Here's how the part is built. I have some questions about the finished solid (model axes, mm). Give positions to 0.01 mm unless a question says otherwise; leave off trailing zeros. Loops run counter-clockwise (first coordinate to the right, second up) from the corner with the lowest first, then second, coordinate; pieces in that order, holes last.
Q1. I need wall thicknesses on line 1 (X direction, y = 6.75, z = 0); line 2 (Z direction, x = 200, y = 12); line 3 (Z direction, x = 107, y = 14.25). Which ranges of each line are inside material? Lowest first, please.
Q2. If we section it at B-B (x = 59.5): Please give me the cut outline in (y, z), plus the area to 3 significant figures.
Q3. If we section it at C-C (y = 13): Please give me the cut outline in (x, z), plus the area to 3 significant figures.
Q4. If we section it at A-A (z = -12.5): Please give me the cut outline in (x, y).
Q5. Will this pin go through, and if not, where does the flat tip stop? P1, Ø12, axis at x = -284.5, z = 59.5, coming from the -Y side.
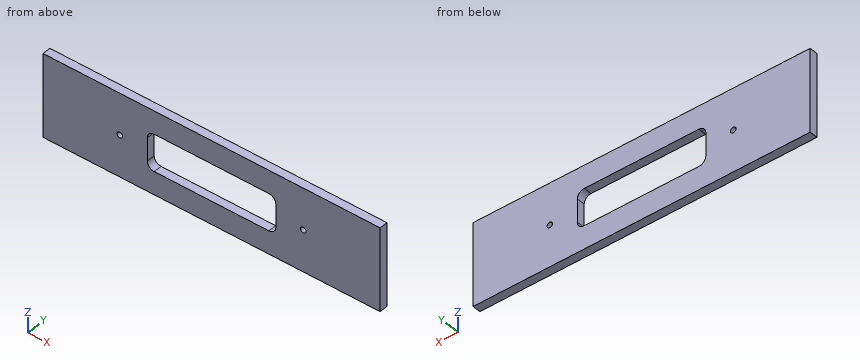
from build123d import *

# Parameters (mm, degrees)
SKETCH1_W           = 735
SKETCH1_H           = 180
BOSS_EXTRUDE1_DEPTH = 18
SKETCH2_R           = 6
CUT_EXTRUDE1_DEPTH  = 60


with BuildPart() as part:
    # Sketch1 → Boss-Extrude1 (new body)
    with BuildSketch(Plane(origin=(0, 0, 0), x_dir=(1, 0, 0), z_dir=(0, 1, 0))):
        Rectangle(SKETCH1_W, SKETCH1_H)
    extrude(amount=BOSS_EXTRUDE1_DEPTH)

    # Sketch2 → Cut-Extrude1 (cut)
    with BuildSketch(Plane(origin=(0, 18, 0), x_dir=(1, 0, 0), z_dir=(0, 1, 0))):
        with Locations((-200, 0)):
            Circle(SKETCH2_R)
        with Locations((200, 0)):
            Circle(SKETCH2_R)
        with BuildLine():
            Line((-125, -40), (125, -40))
            ThreePointArc((125, -40), (135.606601718, -35.606601718), (140, -25))
            Line((140, -25), (140, 25))
            ThreePointArc((140, 25), (135.606601718, 35.606601718), (125, 40))
            Line((125, 40), (-125, 40))
            ThreePointArc((-125, 40), (-135.606601718, 35.606601718), (-140, 25))
            Line((-140, 25), (-140, -25))
            ThreePointArc((-140, -25), (-135.606601718, -35.606601718), (-125, -40))
        make_face()
    extrude(amount=-CUT_EXTRUDE1_DEPTH, mode=Mode.SUBTRACT)


solid = part.part
Check sheet entries:
1. line 1: x = -367.5 to -206, -194 to -140, 140 to 194, 206 to 367.5
1. line 2: z = -90 to -6, 6 to 90
1. line 3: z = -90 to -40, 40 to 90
2. outline: (0, -90) - (18, -90) - (18, -40) - (0, -40) - close; (0, 40) - (18, 40) - (18, 90) - (0, 90) - close
2. area: 1,800 mm2
3. outline: (-367.5, -90) - (367.5, -90) - (367.5, 90) - (-367.5, 90) - close; hole circle Ø12 at (-200, 0); hole (-140, -25) arc R15 ccw to (-125, -40) - (125, -40) arc R15 ccw to (140, -25) - (140, 25) arc R15 ccw to (125, 40) - (-125, 40) arc R15 ccw to (-140, 25) - close; hole circle Ø12 at (200, 0)
3. area: 110,000 mm2
4. outline: (-367.5, 0) - (-140, 0) - (-140, 18) - (-367.5, 18) - close; (140, 0) - (367.5, 0) - (367.5, 18) - (140, 18) - close
5. P1: stops at y = 0
